Source: CAD feature listing. Evaluate the final solid. Frame: model axes, mm. Round coordinates to 2 decimals unless told otherwise and drop trailing zeros. Order: outer loops, then holes, each group sorted by start corner. A loop starts at its lowest first (then second) coordinate and runs counter-clockwise, first axis right, second up. Notation, with made-up numbers: (34, 36) -> (91, 36) arc R20 cw to (91, 46) -> close; hole circle Ø5 at (30.5, -26). An arc over 180 degrees is marked (long way). One line per item, written item: value. Start each with the question number.
1) Section A-A (y = -30.5). Return the cut outline in (x, z).
2) Pin query (flat end, axial travel): P1, Ø0.7, axis at x = 0.5, z = -0.5, coming from the -Y side; P2, Ø1.5, axis at x = -1, y = -35, coming from the -Z side; P3, Ø1.5, axis at y = -8.5, z = -0.5, coming from the +X side. Return the tip coordinate at first contact, or that it passes through.
3) Ray query, L1, parallel to Y at x = 0.15, z = 0.7; L2, parallel to Y at x = 0.85, z = -0.15; L3, parallel to Z at x = 0.1, y = -41.5. Return the intervals inside material, ascending.
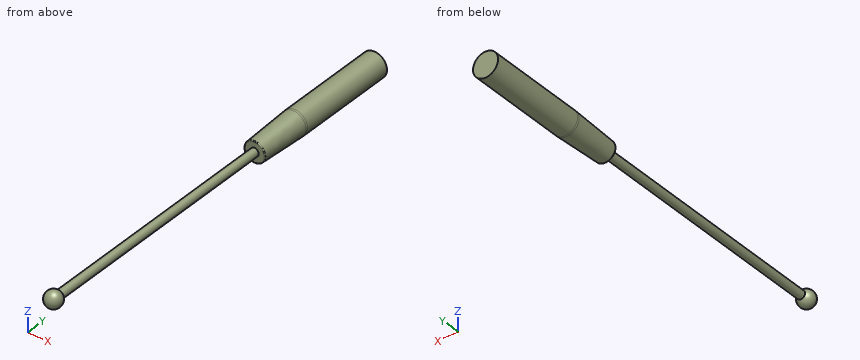
```python
from build123d import *

# Parameters (mm, degrees)
FILLET1_R = 0.1
FILLET2_R = 6


with BuildPart() as part:
    # Sketch1 → Revolve1 (revolve)
    with BuildSketch(Plane.XY):
        with BuildLine():
            Line((0, 0), (1.5, 0))
            Line((1.5, 0), (1.5, -12.5))
            Line((1.5, -12.5), (1.25, -18.682020119))
            Line((1.25, -18.682020119), (0.5, -18.682020119))
            Line((0.5, -18.682020119), (0.5, -49.133974596))
            ThreePointArc((0.5, -49.133974596), (0.965925826, -50.258819045), (0, -51))
            Line((0, -51), (0, 0))
        make_face()
    revolve(axis=Axis((0, -1574.891797032, 0), (0, 1, 0)))

    # Fillet1
    fillet1_edges = [part.edges().sort_by_distance(p)[0] for p in [
        (-1.25, -18.682020119, 0),
    ]]
    fillet(fillet1_edges, radius=FILLET1_R)

    # Fillet2
    # the kernel refuses this fillet: 6 mm, written as the material it takes off along each edge
    with BuildSketch(Plane(origin=(0, -12.5, 0), x_dir=(1, 0, 0), z_dir=(0, 0, 1))) as fillet2_piece_1:
        with BuildLine():
            CenterArc((1.5 - FILLET2_R, FILLET2_R * 0.0202116676517), FILLET2_R, 357.684228799, 2.315771201)
            Line((1.5, FILLET2_R * 0.0202116676517), (1.5, 0))
            Line((1.5, 0), (1.5 - FILLET2_R * 0.000816689391513, -FILLET2_R * 0.0201951609972))
        make_face()
    revolve(axis=Axis((0, -12.5, 0), (0, 1, 0)), mode=Mode.SUBTRACT)


solid = part.part
```
Findings:
1. outline: circle Ø1 at (0, 0)
2. P1: y = -50.93
2. P2: z = -0.43
2. P3: x = 1.5
3. L1: -50.7 to -49.3, -18.68 to 0
3. L2: -50.5 to -49.5, -18.68 to 0
3. L3: -0.49 to 0.49
